Here's how the part is built. I have some questions about the finished solid (model axes, mm). A direction names the side the tool comes from. Give positions to 0.01 mm unless a question says otherwise; leave off trailing zeros. Loops run counter-clockwise (first coordinate to the right, second up) from the corner with the lowest first, then second, coordinate; pieces in that order, holes last. Notation, with made-up numbers: (10, -22.75) -> (23, -22.75) arc R16 ccw to (23, -15.75) -> close; hole circle Ø7 at (71, 12.25). An arc over 180 degrees is marked (long way). Answer in a Markdown table with one row per item. Add a question column.
Item 1: If we section it at B-B (y = 6.5): Write out the boundary of the cut face in (x, z), then the cut area to 3 significant figures.
Item 2: Which directions (+Z, -Z, +X, -X, +Y, -Y) give clear straight access to the entire face, cutting with the end or side of a thin tool? Please do faces 3 (the face through (0, 16, -29)), 4 (the face through (-1, 0, -1)).
Item 3: If I drill on line 1 (Y direction, x = 0, z = 29.65); line 2 (Y direction, x = 0, z = -29.45); line 3 (Z direction, x = -4, y = 10.5), over which ranges is the centre line in solid material (lowest first)?
Item 4: For P1, Ø9, axis at x = 1, y = 14, coming from the -Z side; P2, Ø6, axis at x = -21, z = -50.5, coming from the +Y side; P3, Ø9, axis at x = -4, y = 17, coming from the +Z side; P4, Ø5, axis at y = 4, z = -43, coming from the +X side, each with a flat end and sliding along its axis, tell me the tip position at first contact or that it passes through.
Item 5: If we section it at C-C (z = 50): Write out the boundary of the cut face in (x, y).
Item 6: If we section it at A-A (x = 0): Write out the boundary of the cut face in (y, z), then the cut area to 3 significant figures.
Item 7: We'd pull the mould along X, two halves only. Please class faces 1 (the face through (-0.521, 28.966, 29.507)), 2 (the face through (0, 16, 29)): released by +X, released by -X, zero draft, split by the parting line, or undercut.
Item 8: If we section it at D-D (y = 25): Write out the boundary of the cut face in (x, z).
```python
from build123d import *

# Parameters (mm, degrees)
SKETCH1_W           = 74
SKETCH1_H           = 135
SKETCH1_W_2         = 18
SKETCH1_H_2         = 30
BOSS_EXTRUDE1_DEPTH = 1
BOSS_EXTRUDE2_START = -1
SKETCH2_W           = 18
SKETCH2_H           = 1
BOSS_EXTRUDE2_DEPTH = 31
CUT_EXTRUDE3_REACH  = 99.5
SKETCH5_R           = 4
CUT_EXTRUDE4_REACH  = 40.5
SKETCH6_R           = 1.5
FILLET2_R           = 2


with BuildPart() as part:
    # Sketch1 → Boss-Extrude1 (new body)
    with BuildSketch(Plane(origin=(0, 0, 0), x_dir=(1, 0, 0), z_dir=(0, 1, 0))):
        Rectangle(SKETCH1_W, SKETCH1_H)
        with Locations((0, 44)):
            Rectangle(SKETCH1_W_2, SKETCH1_H_2, mode=Mode.SUBTRACT)
        with Locations((0, -44)):
            Rectangle(SKETCH1_W_2, SKETCH1_H_2, mode=Mode.SUBTRACT)
    extrude(amount=BOSS_EXTRUDE1_DEPTH)

    # Sketch2 → Boss-Extrude2 (add)
    with BuildSketch(Plane(origin=(0, 1, 0), x_dir=(1, 0, 0), z_dir=(0, 1, 0)).offset(BOSS_EXTRUDE2_START)):
        with Locations((0, 29.5)):
            Rectangle(SKETCH2_W, SKETCH2_H)
        with Locations((0, -29.5)):
            Rectangle(SKETCH2_W, SKETCH2_H)
    extrude(amount=BOSS_EXTRUDE2_DEPTH)

    # Sketch5 → Cut-Extrude3 (cut, up to next)
    with BuildSketch(Plane.XY.offset(30), mode=Mode.PRIVATE) as cut_extrude3_sk1:
        with Locations((0, 25)):
            Circle(SKETCH5_R)
    cut_extrude3_tool1 = extrude(cut_extrude3_sk1.sketch, amount=-CUT_EXTRUDE3_REACH, mode=Mode.PRIVATE) & part.part
    add(cut_extrude3_tool1.solids().sort_by_distance((0, 25, 30))[0], mode=Mode.SUBTRACT)

    # Sketch6 → Cut-Extrude4 (cut, up to next)
    with BuildSketch(Plane.XY.offset(-29), mode=Mode.PRIVATE) as cut_extrude4_sk1:
        with Locations((0, 25)):
            Circle(SKETCH6_R)
    cut_extrude4_tool1 = extrude(cut_extrude4_sk1.sketch, amount=-CUT_EXTRUDE4_REACH, mode=Mode.PRIVATE) & part.part
    add(cut_extrude4_tool1.solids().sort_by_distance((0, 25, -29))[0], mode=Mode.SUBTRACT)

    # Fillet2
    fillet2_edges = [part.edges().sort_by_distance(p)[0] for p in [
        (9, 0.5, -59),
        (-9, 0.5, -59),
        (-9, 0.5, 59),
        (9, 0.5, 59),
        (-9, 31, -29.5),
        (9, 31, -29.5),
        (-9, 31, 29.5),
        (9, 31, 29.5),
        (37, 0.5, 67.5),
        (-37, 0.5, 67.5),
        (-37, 0.5, -67.5),
        (37, 0.5, -67.5),
    ]]
    fillet(fillet2_edges, radius=FILLET2_R)


solid = part.part
```
Recorded:
| question | item | result |
|---|---|---|
| 1 | outline | (-9, -30) -> (9, -30) -> (9, -29) -> (-9, -29) -> close; (-9, 29) -> (9, 29) -> (9, 30) -> (-9, 30) -> close |
| 1 | area | 36.0 mm^2 |
| 2 | face 3 | +X, -X, +Y |
| 2 | face 4 | +Z, -Z, +X, -X, -Y |
| 3 | line 1 | y = 0 to 21, 29 to 31 |
| 3 | line 2 | y = 0 to 23.5, 26.5 to 31 |
| 3 | line 3 | z = -30 to -29, 29 to 30 |
| 4 | P1 | stops at z = -30 |
| 4 | P2 | stops at y = 1 |
| 4 | P3 | stops at z = 30 |
| 4 | P4 | passes through |
| 5 | outline | (-37, 0) -> (-9, 0) -> (-9, 1) -> (-37, 1) -> close; (9, 0) -> (37, 0) -> (37, 1) -> (9, 1) -> close |
| 6 | outline | (0, -67.5) -> (1, -67.5) -> (1, -59) -> (0, -59) -> close; (0, -30) -> (23.5, -30) -> (23.5, -29) -> (1, -29) -> (1, 29) -> (21, 29) -> (21, 30) -> (0, 30) -> close; (0, 59) -> (1, 59) -> (1, 67.5) -> (0, 67.5) -> close; (26.5, -30) -> (31, -30) -> (31, -29) -> (26.5, -29) -> close; (29, 29) -> (31, 29) -> (31, 30) -> (29, 30) -> close |
| 6 | area | 126 mm^2 |
| 7 | face 1 | undercut |
| 7 | face 2 | zero draft |
| 8 | outline | (-9, -30) -> (-1.5, -30) -> (-1.5, -29) -> (-9, -29) -> close; (-9, 29) -> (-4, 29) -> (-4, 30) -> (-9, 30) -> close; (1.5, -30) -> (9, -30) -> (9, -29) -> (1.5, -29) -> close; (4, 29) -> (9, 29) -> (9, 30) -> (4, 30) -> close |
